```python
from build123d import *

# Parameters (mm, degrees)
SKETCH2_R           = 5.5
SKETCH2_R_2         = 1.750005389
SKETCH2_R_3         = 1.749978063
SKETCH2_R_4         = 1.749044057
BOSS_EXTRUDE1_DEPTH = 5
BOSS_EXTRUDE2_START = 6
SKETCH3_R           = 1
SKETCH3_W           = 23
SKETCH3_H           = 11.999999553
BOSS_EXTRUDE2_DEPTH = 6
SKETCH4_W           = 8.00000038
SKETCH4_H           = 26
BOSS_EXTRUDE3_DEPTH = 18
BOSS_EXTRUDE4_DEPTH = 4
FILLET1_R           = 8.5
SKETCH6_R           = 2.5
SKETCH6_R_2         = 1.3
CUT_EXTRUDE1_DEPTH  = 87.192574237


with BuildPart() as part:
    # Sketch2 → Boss-Extrude1 (new body)
    with BuildSketch(Plane.XY):
        with BuildLine():
            Line((6.000000052, -0.218525005), (14.000000432, -0.218525005))
            Line((14.000000432, -0.218525005), (14.000000432, -28.000000864))
            Line((14.000000432, -28.000000864), (14.000000432, -28.50000152))
            ThreePointArc((14.000000432, -28.50000152), (15.025126698, -30.974875254), (17.500000432, -32.00000152))
            Line((17.500000432, -32.00000152), (17.999999225, -32.00000152))
            Line((17.999999225, -32.00000152), (24.343099445, -32.00000152))
            Line((24.343099445, -32.00000152), (24.550253068, -32.00000152))
            ThreePointArc((24.550253068, -32.00000152), (25.889645081, -32.266423156), (27.025126802, -33.025127786))
            Line((27.025126802, -33.025127786), (27.17160061, -33.171601593))
            Line((27.17160061, -33.171601593), (34.828398377, -40.82839936))
            Line((34.828398377, -40.82839936), (34.974872184, -40.974873168))
            ThreePointArc((34.974872184, -40.974873168), (36.110353905, -41.733577798), (37.449745919, -41.999999434))
            Line((37.449745919, -41.999999434), (37.656899542, -41.999999434))
            Line((37.656899542, -41.999999434), (40.399998426, -41.999999434))
            Line((40.399998426, -41.999999434), (40.899999082, -41.999999434))
            ThreePointArc((40.899999082, -41.999999434), (43.374872816, -43.0251257), (44.399999082, -45.499999434))
            Line((44.399999082, -45.499999434), (44.399999082, -46.000000089))
            Line((44.399999082, -46.000000089), (44.399999082, -57.999998331))
            Line((44.399999082, -57.999998331), (44.399999082, -58.499998987))
            ThreePointArc((44.399999082, -58.499998987), (43.374872816, -60.974872721), (40.899999082, -61.999998987))
            Line((40.899999082, -61.999998987), (40.399998426, -61.999998987))
            Line((40.399998426, -61.999998987), (38.140699267, -61.999998987))
            Line((38.140699267, -61.999998987), (37.873109304, -61.999998987))
            ThreePointArc((37.873109304, -61.999998987), (36.221600534, -62.414141118), (34.960925686, -63.558559682))
            Line((34.960925686, -63.558559682), (34.812498838, -63.781201839))
            Line((34.812498838, -63.781201839), (27.187500149, -75.21879673))
            Line((27.187500149, -75.21879673), (27.039073301, -75.441438887))
            ThreePointArc((27.039073301, -75.441438887), (25.778398453, -76.585857451), (24.126889683, -76.999999583))
            Line((24.126889683, -76.999999583), (23.859299719, -76.999999583))
            Line((23.859299719, -76.999999583), (12.140699662, -76.999999583))
            Line((12.140699662, -76.999999583), (11.893097313, -76.999999583))
            ThreePointArc((11.893097313, -76.999999583), (10.313829571, -76.62344534), (9.074378953, -75.574807238))
            Line((9.074378953, -75.574807238), (8.814488373, -75.22173434))
            Line((8.814488373, -75.22173434), (0.671799004, -63.007697463))
            Line((0.671799004, -63.007697463), (0.587823763, -62.881734572))
            ThreePointArc((0.587823763, -62.881734572), (0.150177853, -61.954528538), (0, -60.940284196))
            Line((0, -60.940284196), (0, -60.78889966))
            Line((0, -60.78889966), (0, -44.708199799))
            Line((0, -44.708199799), (0, -44.517187636))
            ThreePointArc((0, -44.517187636), (0.230396061, -43.268312109), (0.891251475, -42.183857155))
            Line((0.891251475, -42.183857155), (1.018580049, -42.041499168))
            Line((1.018580049, -42.041499168), (4.981420003, -37.610899657))
            Line((4.981420003, -37.610899657), (5.108748578, -37.46854167))
            ThreePointArc((5.108748578, -37.46854167), (5.769603991, -36.384086716), (6.000000052, -35.135211189))
            Line((6.000000052, -35.135211189), (6.000000052, -34.944299609))
            Line((6.000000052, -34.944299609), (6.000000052, -0.218525005))
        make_face()
        with Locations((31.910091824, -52.001420952)):
            Circle(SKETCH2_R, mode=Mode.SUBTRACT)
        with Locations((22.999980116, -71.999985367)):
            Circle(SKETCH2_R_2, mode=Mode.SUBTRACT)
        with Locations((13.000012747, -72.0000118)):
            Circle(SKETCH2_R_3, mode=Mode.SUBTRACT)
        with Locations((4.995051671, -52.002868251)):
            Circle(SKETCH2_R_4, mode=Mode.SUBTRACT)
    extrude(amount=BOSS_EXTRUDE1_DEPTH)

    # Sketch3 → Boss-Extrude2 (add)
    with BuildSketch(Plane(origin=(0, 0, 0), x_dir=(-1, 0, 0), z_dir=(0, 0, -1)).offset(BOSS_EXTRUDE2_START)):
        with BuildLine():
            Line((-37.873109304, -61.999998987), (-40.899999082, -61.999998987))
            ThreePointArc((-40.899999082, -61.999998987), (-43.374872816, -60.974872721), (-44.399999082, -58.499998987))
            Line((-44.399999082, -58.499998987), (-44.399999082, -45.499999434))
            ThreePointArc((-44.399999082, -45.499999434), (-43.374872816, -43.0251257), (-40.899999082, -41.999999434))
            Line((-40.899999082, -41.999999434), (-37.449745919, -41.999999434))
            Line((-37.449745919, -41.999999434), (-17.500000432, -41.999999434))
            ThreePointArc((-17.500000432, -41.999999434), (-15.025126698, -40.974873168), (-14.000000432, -38.499999434))
            Line((-14.000000432, -38.499999434), (-14.000000432, -0.218525005))
            Line((-14.000000432, -0.218525005), (-6.000000052, -0.218525005))
            Line((-6.000000052, -0.218525005), (-6.000000052, -41.999999434))
            Line((-6.000000052, -41.999999434), (-7.399999082, -41.999999434))
            ThreePointArc((-7.399999082, -41.999999434), (-8.814212644, -42.585785871), (-9.399999082, -43.999999434))
            Line((-9.399999082, -43.999999434), (-9.399999082, -58.499998987))
            ThreePointArc((-9.399999082, -58.499998987), (-10.425125348, -60.974872721), (-12.899999082, -61.999998987))
            Line((-12.899999082, -61.999998987), (-37.873109304, -61.999998987))
        make_face()
        with Locations((-40.699999082, -51.99999921)):
            Circle(SKETCH3_R, mode=Mode.SUBTRACT)
        with Locations(Location((-13.099999082, -51.99999921, 0), (0, 0, 180))):
            Circle(SKETCH3_R, mode=Mode.SUBTRACT)
        with Locations((-26.899999082, -51.999999211)):
            Rectangle(SKETCH3_W, SKETCH3_H, mode=Mode.SUBTRACT)
    extrude(amount=-BOSS_EXTRUDE2_DEPTH)

    # Sketch4 → Boss-Extrude3 (add)
    with BuildSketch(Plane(origin=(0, 0, -6), x_dir=(-1, 0, 0), z_dir=(0, 0, -1))):
        with Locations((-10.000000242, -13.218525005)):
            Rectangle(SKETCH4_W, SKETCH4_H)
    extrude(amount=BOSS_EXTRUDE3_DEPTH)

    # Sketch5 → Boss-Extrude4 (add, symmetric)
    with BuildSketch(Plane.ZY.offset(-10.000000242)):
        Polygon((-24, -26.218525005), (-6, -41.999999434), (-6, -26.218525005), align=None)
    extrude(amount=BOSS_EXTRUDE4_DEPTH, both=True)

    # Fillet1
    fillet1_edges = [part.edges().sort_by_distance(p)[0] for p in [
        (10.000000242, -0.218525005, 5),
        (10.000000242, -26.218525005, -24),
        (10.000000242, -0.218525005, -24),
    ]]
    fillet(fillet1_edges, radius=FILLET1_R)

    # Sketch6 → Cut-Extrude1 (cut, through all)
    with BuildSketch(Plane(origin=(14.000000432, 0, 0), x_dir=(0, 0, -1), z_dir=(1, 0, 0))):
        with Locations(Location((9.49999962, -14.218525005, 0), (0, 0, 90))):
            Circle(SKETCH6_R)
        with Locations(Location((9.5, -9.518525005, 0), (0, 0, 90))):
            Circle(SKETCH6_R_2)
        with Locations((9.5, -18.918525005)):
            Circle(SKETCH6_R_2)
    extrude(amount=-CUT_EXTRUDE1_DEPTH, mode=Mode.SUBTRACT)


solid = part.part
```
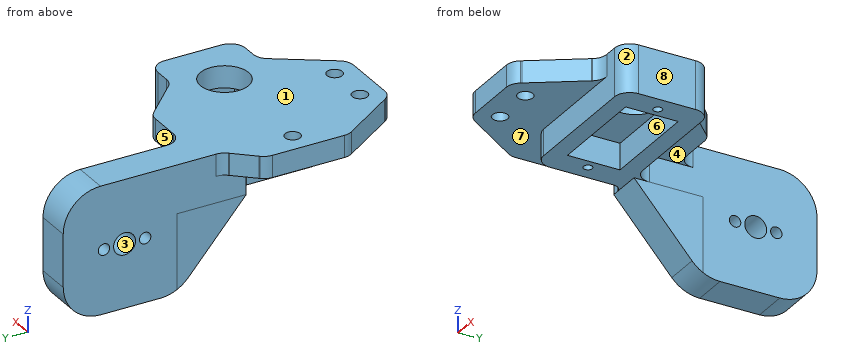
Geometry check sheet. Reference: the model listing, model coordinates, mm. Face numbers are marked on the shaded views. A direction names the side the tool comes from. Give positions to 0.01 mm unless a question says otherwise; leave off trailing zeros. Write each loop counter-clockwise with the first axis right and the second up, starting at its lowest first coordinate (ties: lowest second). Pieces come first, ordered by that corner, then holes.
1) Section check C-C, the plane z = 1.25. State how many separate pieces and enclosed holes the cut face has, and give its area (3 significant figures).
2) Release check for a two-part mould opening along Z. For the marked faces 1, 2, 3 and 4 record: pulls with the +Z half, pulls with the -Z half, needs draft (parallel to the pull), parting line crosses it, or undercut.
3) Gauge pin test, flat ends, axial feed: pin 1 (1 mm diameter, centred on x = 37, z = 0.5, fed in from +Y); pin 2 (3 mm diameter, centred on x = 40.7, y = -52, fed in from -Z); pin 3 (10 mm diameter, centred on y = -19.5, z = -16, fed in from -X); pin 4 (6.5 mm diameter, centred on x = 31.91, y = -52, fed in from +Z). Record the tip position at first contact, or that the pin passes through.
4) Material ranges on L1, parallel to X at y = -55, z = -5.25; L2, parallel to Y at x = 33.5, z = -5.25; L3, parallel to X at y = -51, z = 1, recorded low to high.
5) Section check A-A, the plane z = -9.5. Record the boundary of the cut face in (x, y), and give its area (3 significant figures).
6) Access from +Z, -Z, +X, -X, +Y, -Y to the whole of each face (thin tool, end or side, straight path). Record for the marked faces 5, 6, 7 and 8.
7) Section check B-B, the plane x = 32. Record the boundary of the cut face in (y, z), and give its area (3 significant figures).
Computed:
1. separate pieces: 1
1. enclosed holes: 4
1. area: 1,660 mm2
2. face 1: pulls with the +Z half
2. face 2: needs draft
2. face 3: undercut
2. face 4: pulls with the -Z half
3. pin 1: stops at y = -41.87
3. pin 2: stops at z = -6
3. pin 3: stops at x = 6
3. pin 4: passes through
4. L1: x = 9.4 to 15.4, 38.4 to 44.4
4. L2: y = -62 to -58, -46 to -42
4. L3: x = 0 to 3.56, 6.43 to 26.5, 37.32 to 44.4
5. outline: (6, -38.93) - (14, -38.93) - (14, -20.22) - (6, -20.22) - close; (6, -17.62) - (14, -17.62) - (14, -16.72) - (6, -16.72) - close; (6, -11.72) - (14, -11.72) - (14, -10.82) - (6, -10.82) - close; (6, -8.22) - (14, -8.22) - (14, -0.22) - (6, -0.22) - close
5. area: 228 mm2
6. face 5: +Z, -Z, +X, +Y
6. face 6: -Z
6. face 7: -Z, -X, -Y
6. face 8: +Z, -Z, +X, +Y, -Y
7. outline: (-68, 0) - (-62, 0) - (-62, -6) - (-58, -6) - (-58, 0) - (-57.5, 0) - (-57.5, 5) - (-68, 5) - close; (-46.5, 0) - (-46, 0) - (-46, -6) - (-42, -6) - (-42, 0) - (-38, 0) - (-38, 5) - (-46.5, 5) - close
7. area: 143 mm2
